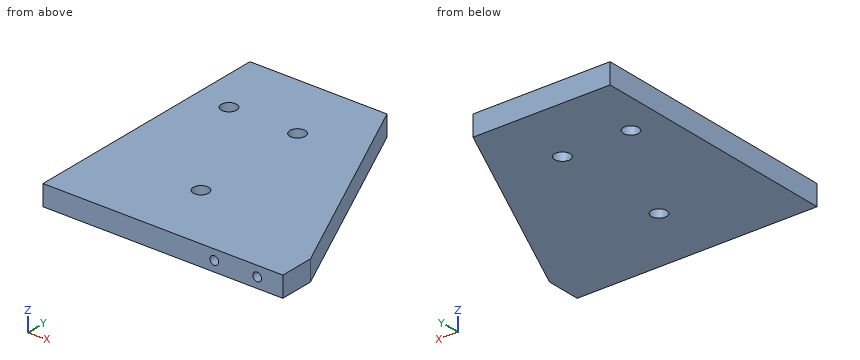
```python
from build123d import *

# Parameters (mm, degrees)
BOSS_EXTRUDE1_DEPTH     = 12
CUT_EXTRUDE1_DEPTH      = 206.533452265
CUT_EXTRUDE1_DEPTH_BACK = 206.533452265
SKETCH2_R               = 4.5
SKETCH3_R               = 2.5
CUT_EXTRUDE3_DEPTH      = 15


with BuildPart() as part:
    # Sketch1 → Boss-Extrude1 (new body)
    with BuildSketch(Plane.XY):
        Polygon((0, 0), (140, 0), (140, 20), (80, 150), (0, 150), align=None)
    extrude(amount=BOSS_EXTRUDE1_DEPTH)

    # Sketch2 → Cut-Extrude1 (cut, two sides: drawn at the far end of the back side and taken through both)
    with BuildSketch(Plane.XY.offset(-CUT_EXTRUDE1_DEPTH_BACK)):
        with Locations((20, 110)):
            Circle(SKETCH2_R)
        with Locations((60, 110)):
            Circle(SKETCH2_R)
        with Locations((60, 40)):
            Circle(SKETCH2_R)
    extrude(amount=CUT_EXTRUDE1_DEPTH + CUT_EXTRUDE1_DEPTH_BACK, mode=Mode.SUBTRACT)

    # Sketch3 → Cut-Extrude3 (cut)
    with BuildSketch(Plane(origin=(0, 0, 0), x_dir=(1, 0, 0), z_dir=(0, 1, 0))):
        with Locations(Location((100, -6, 0), (0, 0, 270))):
            Circle(SKETCH3_R)
        with Locations(Location((125, -6, 0), (0, 0, 270))):
            Circle(SKETCH3_R)
    extrude(amount=CUT_EXTRUDE3_DEPTH, mode=Mode.SUBTRACT)


solid = part.part
```
Check sheet for the modelled part. Datum: model origin and axes. Units: mm. Round coordinates to 2 decimals unless told otherwise and drop trailing zeros. Order: outer loops, then holes, each group sorted by start corner. A loop starts at its lowest first (then second) coordinate and runs counter-clockwise, first axis right, second up.
1) Scan lines: line 1 (X direction, y = 5.5, z = 6); line 2 (X direction, y = 109, z = 2.5); line 3 (Y direction, x = 57.5, z = 1.5). Record each from-to range of solid material in increasing order.
2) Section check D-D (x = 125). Record the boundary of the cut face in (y, z), and give its area (3 significant figures).
3) Section check B-B (y = 110). Record the boundary of the cut face in (x, z), and give its area (3 significant figures).
4) Section check A-A (x = 20). Record the boundary of the cut face in (y, z), and give its area (3 significant figures).
5) Go/stop test with flat-tipped pins: pin 1 Ø4 at (x, z) = (125, 6) entering from -Y; pin 2 Ø6 at (x, z) = (100, 6) entering from +Y. Record where each tip stops, or that it passes through.
6) Section check C-C (z = 6). Record the boundary of the cut face in (x, y), and give its area (3 significant figures).
Result:
1. line 1: x = 0 to 97.5, 102.5 to 122.5, 127.5 to 140
1. line 2: x = 0 to 15.61, 24.39 to 55.61, 64.39 to 98.92
1. line 3: y = 0 to 36.26, 43.74 to 106.26, 113.74 to 150
2. outline: (0, 0) - (52.5, 0) - (52.5, 12) - (0, 12) - (0, 8.5) - (15, 8.5) - (15, 3.5) - (0, 3.5) - close
2. area: 555 mm2
3. outline: (0, 0) - (15.5, 0) - (15.5, 12) - (0, 12) - close; (24.5, 0) - (55.5, 0) - (55.5, 12) - (24.5, 12) - close; (64.5, 0) - (98.46, 0) - (98.46, 12) - (64.5, 12) - close
3. area: 966 mm2
4. outline: (0, 0) - (105.5, 0) - (105.5, 12) - (0, 12) - close; (114.5, 0) - (150, 0) - (150, 12) - (114.5, 12) - close
4. area: 1,690 mm2
5. pin 1: stops at y = 15
5. pin 2: stops at y = 113.17
6. outline: (0, 0) - (97.5, 0) - (97.5, 15) - (102.5, 15) - (102.5, 0) - (122.5, 0) - (122.5, 15) - (127.5, 15) - (127.5, 0) - (140, 0) - (140, 20) - (80, 150) - (0, 150) - close; hole circle Ø9 at (20, 110); hole circle Ø9 at (60, 40); hole circle Ø9 at (60, 110)
6. area: 16,800 mm2
